```python
from build123d import *

# Parameters (mm, degrees)
SKETCH1_W           = 64
SKETCH1_H           = 76
TOP_DEPTH           = 2
SKETCH2_W           = 59.8
SKETCH2_H           = 71.8
BOSS_EXTRUDE2_DEPTH = 3
SKETCH3_W           = 10.5
SKETCH3_H           = 10.5
CUT_EXTRUDE1_DEPTH  = 6
SKETCH10_W          = 25.7
SKETCH10_H          = 27
CUT_EXTRUDE8_DEPTH  = 3
SKETCH11_W          = 7
SKETCH11_H          = 8
CUT_EXTRUDE9_DEPTH  = 1
SKETCH6_W           = 30
SKETCH6_H           = 25.4
CUT_EXTRUDE4_DEPTH  = 6
SKETCH7_R           = 1.15
BOSS_EXTRUDE3_DEPTH = 4.7
SKETCH8_W           = 40.8
SKETCH8_H           = 30.6
CUT_EXTRUDE6_DEPTH  = 4.7
SKETCH9_W           = 6.8
SKETCH9_H           = 15
CUT_EXTRUDE7_DEPTH  = 4.7
FILLET2_R           = 20
FILLET3_START       = 0.3
FILLET3_DEPTH       = 5.7
FILLET3_START_2     = 1
FILLET3_2_DEPTH     = 11
SKETCH14_R          = 1.15
BOSS_EXTRUDE4_DEPTH = 4.5
SKETCH12_W          = 11.9
SKETCH12_H          = 8
CUT_EXTRUDE10_DEPTH = 4
FILLET4_R           = 20
FILLET5_R           = 5


with BuildPart() as part:
    # Sketch1 → Top (new body)
    with BuildSketch(Plane(origin=(0, 0, 0), x_dir=(1, 0, 0), z_dir=(0, 1, 0))):
        Rectangle(SKETCH1_W, SKETCH1_H)
    extrude(amount=TOP_DEPTH)

    # Sketch2 → Boss-Extrude2 (add)
    with BuildSketch(Plane(origin=(0, 2, 0), x_dir=(1, 0, 0), z_dir=(0, 1, 0))):
        Rectangle(SKETCH2_W, SKETCH2_H)
    extrude(amount=BOSS_EXTRUDE2_DEPTH)

    # Sketch3 → Cut-Extrude1 (cut)
    with BuildSketch(Plane(origin=(0, 5, 0), x_dir=(1, 0, 0), z_dir=(0, 1, 0))):
        with Locations((-14.15, 20.15)):
            Rectangle(SKETCH3_W, SKETCH3_H)
    extrude(amount=-CUT_EXTRUDE1_DEPTH, mode=Mode.SUBTRACT)

    # Sketch10 → Cut-Extrude8 (cut)
    with BuildSketch(Plane(origin=(0, 5, 0), x_dir=(1, 0, 0), z_dir=(0, 1, 0))):
        with Locations((-14.15, 20.15)):
            Rectangle(SKETCH10_W, SKETCH10_H)
    extrude(amount=-CUT_EXTRUDE8_DEPTH, mode=Mode.SUBTRACT)

    # Sketch11 → Cut-Extrude9 (cut)
    with BuildSketch(Plane(origin=(0, 2, 0), x_dir=(1, 0, 0), z_dir=(0, 1, 0))):
        with Locations((-22.9, 20.15)):
            Rectangle(SKETCH11_W, SKETCH11_H)
        with Locations((-5.4, 20.15)):
            Rectangle(SKETCH11_W, SKETCH11_H)
    extrude(amount=-CUT_EXTRUDE9_DEPTH, mode=Mode.SUBTRACT)

    # Sketch6 → Cut-Extrude4 (cut)
    with BuildSketch(Plane(origin=(0, 5, 0), x_dir=(1, 0, 0), z_dir=(0, 1, 0))):
        with Locations((6.6, -17.5)):
            Rectangle(SKETCH6_W, SKETCH6_H)
    extrude(amount=-CUT_EXTRUDE4_DEPTH, mode=Mode.SUBTRACT)

    # Sketch7 → Boss-Extrude3 (add)
    with BuildSketch(Plane(origin=(0, 5, 0), x_dir=(1, 0, 0), z_dir=(0, 1, 0))):
        with Locations((-11.5, -4.5)):
            Circle(SKETCH7_R)
        with Locations((-11.5, -30.5)):
            Circle(SKETCH7_R)
        with Locations((24.7, -30.5)):
            Circle(SKETCH7_R)
        with Locations((24.7, -4.5)):
            Circle(SKETCH7_R)
    extrude(amount=-BOSS_EXTRUDE3_DEPTH)

    # Sketch8 → Cut-Extrude6 (cut)
    with BuildSketch(Plane(origin=(0, 5, 0), x_dir=(1, 0, 0), z_dir=(0, 1, 0))):
        with Locations((6.6, -17.5)):
            Rectangle(SKETCH8_W, SKETCH8_H)
    extrude(amount=-CUT_EXTRUDE6_DEPTH, mode=Mode.SUBTRACT)

    # Sketch9 → Cut-Extrude7 (cut)
    with BuildSketch(Plane(origin=(0, 5, 0), x_dir=(1, 0, 0), z_dir=(0, 1, 0))):
        with Locations((6.6, 5.3)):
            Rectangle(SKETCH9_W, SKETCH9_H)
    extrude(amount=-CUT_EXTRUDE7_DEPTH, mode=Mode.SUBTRACT)

    # Fillet2
    # the kernel refuses this fillet: 20 mm, written as the material it adds along each edge
    with BuildSketch(Plane(origin=(3.2, 0.3, -12.8), x_dir=(0, 0, 1), z_dir=(1, 0, 0))) as fillet2_piece_1:
        with BuildLine():
            CenterArc((12.880605576, -20), FILLET2_R, 90, 40.093007985)
            Line((0, -4.7), (0, 0))
            Line((0, 0), (12.880605576, 0))
        make_face()
    extrude(amount=6.8)

    # Fillet3: read off the stored shape, not the designer's step
    # Fillet3 outline → Fillet3 (cut)
    with BuildSketch(Plane(origin=(0, 0, 0), x_dir=(1, 0, 0), z_dir=(0, 1, 0)).offset(FILLET3_START)):
        with BuildLine():
            ThreePointArc((15, -2.2), (11.464466094, -0.735533906), (10, 2.8))
            Line((10, 2.8), (10, -2.2))
            Line((10, -2.2), (15, -2.2))
        make_face()
        with BuildLine():
            ThreePointArc((3.2, 2.8), (1.735533906, -0.735533906), (-1.8, -2.2))
            Line((-1.8, -2.2), (3.2, -2.2))
            Line((3.2, -2.2), (3.2, 2.8))
        make_face()
    extrude(amount=FILLET3_DEPTH, mode=Mode.SUBTRACT)

    # Fillet3 2 outline → Fillet3 2 (add)
    with BuildSketch(Plane.YZ.offset(FILLET3_START_2)):
        with BuildLine():
            Line((0.3, 0.080605576), (0.3, -2.8))
            Line((0.3, -2.8), (0.508534377, -2.8))
            ThreePointArc((0.508534377, -2.8), (0.35220172, -1.363466364), (0.3, 0.080605576))
        make_face()
    extrude(amount=FILLET3_2_DEPTH)

    # Sketch14 → Boss-Extrude4 (add)
    with BuildSketch(Plane(origin=(0, 0.3, 0), x_dir=(1, 0, 0), z_dir=(0, 1, 0))):
        with Locations(Location((-11.5, -4.5, 0), (0, 0, 270))):
            Circle(SKETCH14_R)
        with Locations(Location((24.7, -4.5, 0), (0, 0, 90))):
            Circle(SKETCH14_R)
        with Locations(Location((24.7, -30.5, 0), (0, 0, 270))):
            Circle(SKETCH14_R)
        with Locations(Location((-11.5, -30.5, 0), (0, 0, 90))):
            Circle(SKETCH14_R)
    extrude(amount=BOSS_EXTRUDE4_DEPTH)

    # Sketch12 → Cut-Extrude10 (cut)
    with BuildSketch(Plane(origin=(0, 5, 0), x_dir=(1, 0, 0), z_dir=(0, 1, 0))):
        with Locations((4.05, 20.15)):
            Rectangle(SKETCH12_W, SKETCH12_H)
    extrude(amount=-CUT_EXTRUDE10_DEPTH, mode=Mode.SUBTRACT)

    # Fillet4
    # the kernel refuses this fillet: 20 mm, written as the material it adds along each edge
    with BuildSketch(Plane(origin=(10, 1, -54.15), x_dir=(-1, 0, 0), z_dir=(0, 0, 1))) as fillet4_piece_1_section:
        with BuildLine():
            CenterArc((12, -20), FILLET4_R, 90, 36.869897646)
            Line((0, -4), (0, 0))
            Line((0, 0), (12, 0))
        make_face()
    fillet4_piece_1 = extrude(amount=38, mode=Mode.PRIVATE)
    fillet4_piece_1 = split(fillet4_piece_1, bisect_by=Plane(origin=(10, 1, -35.9), z_dir=(0, 0, 1)), keep=Keep.TOP, mode=Mode.PRIVATE)
    add(fillet4_piece_1)

    # Fillet5
    fillet5_edges = [part.edges().sort_by_distance(p)[0] for p in [
        (-1.3, 3.5, -24.15),
        (-1.3, 3.5, -16.15),
    ]]
    fillet(fillet5_edges, radius=FILLET5_R)


solid = part.part
```
The listing builds one solid part. Answer for the finished solid, in the listing's coordinates (mm). A direction names the side the tool comes from. Coordinates: 2 decimals unless noted, no trailing zeros. Loops run counter-clockwise (first coordinate to the right, second up) from the corner with the lowest first, then second, coordinate; pieces in that order, holes last. Notation, with made-up numbers: (27.5, 41.25) - (51.5, 41.25) arc R21 ccw to (51.5, 74.25) - close; hole circle Ø6 at (70.25, 62.5). An arc over 180 degrees is marked (long way). Use a Markdown table: item, result. Add a question column.
1) Find the intervals of material crossed by line 1 (X direction, y = 3.7, z = -10.5); line 2 (Z direction, x = -2.5, y = 2.7); line 3 (X direction, y = 2.6, z = -32.5), in increasing order.
2) For faces 1 (the flat face through (-5, 1, -20)), 2 (the flat face through (0, 1, 38)), 3 (the flat face through (-14, 1, -14.9)), 4 (the flat face through (0, 3, 35.9)), determine the directions among +Z, -Z, +X, -X, +Y, -Y from which every point of the face is accessible in a straight line to the end or side of a thin tool.
3) The part is cut by section C-C, the plane y = 3.5. Give the vertices of the cut face in (x, z), and give its area (3 significant figures).
4) Given pin 1 (2.5 mm diameter, centred on x = -11, z = 5, fed in from +Y); pin 2 (1.3 mm diameter, centred on y = 3, z = -6, fed in from -X); pin 3 (2 mm diameter, centred on x = 18, y = 4.5, fed in from +Z), each flat-ended and moving along its own axis, determine where each tip first touches the part or whether it passes through.
5) The part is cut by section D-D, the plane x = 24.7. Give the vertices of the cut face in (y, z), and give its area (3 significant figures).
6) The part is cut by section B-B, the plane z = -22. Give the vertices of the cut face in (x, y), and give its area (3 significant figures).
7) The part is cut by section A-A, the plane x = -4. Give the vertices of the cut face in (y, z), and give its area (3 significant figures).
Here are the results:
| question | item | result |
|---|---|---|
| 1 | line 1 | x = -29.9 to -27, -1.3 to 3.2, 10 to 29.9 |
| 1 | line 2 | z = -35.9 to -33.65, -6.65 to 2.2, 32.8 to 35.9 |
| 1 | line 3 | x = -29.9 to -27, -1.3 to 29.9 |
| 2 | face 1 | +Y |
| 2 | face 2 | +Z, +X, -X, +Y, -Y |
| 2 | face 3 | +Y, -Y |
| 2 | face 4 | +Z, +X, -X, +Y |
| 3 | outline | (-29.9, -35.9) - (29.9, -35.9) - (29.9, 35.9) - (-29.9, 35.9) - close; circle Ø2.3 at (-11.5, 4.5); circle Ø2.3 at (-11.5, 30.5); circle Ø2.3 at (24.7, 4.5); circle Ø2.3 at (24.7, 30.5); hole (-27, -33.65) - (-1.3, -33.65) - (-1.3, -29.15) arc R5 cw to (3.7, -24.15) - (7.68, -24.15) - (7.68, -16.15) - (3.7, -16.15) arc R5 cw to (-1.3, -11.15) - (-1.3, -6.65) - (-27, -6.65) - close; hole (-13.8, 2.2) - (-1.8, 2.2) arc R5 cw to (3.2, -2.8) - (3.2, -10.77) - (10, -10.77) - (10, -2.8) arc R5 cw to (15, 2.2) - (27, 2.2) - (27, 32.8) - (-13.8, 32.8) - close |
| 3 | area | 2,190 mm^2 |
| 4 | pin 1 | stops at y = 4.8 |
| 4 | pin 2 | stops at x = -29.9 |
| 4 | pin 3 | stops at z = 35.9 |
| 5 | outline | (0, -38) - (2, -38) - (2, -35.9) - (5, -35.9) - (5, 2.2) - (0.3, 2.2) - (0.3, 3.35) - (4.8, 3.35) - (4.8, 5.65) - (0.3, 5.65) - (0.3, 29.35) - (4.8, 29.35) - (4.8, 31.65) - (0.3, 31.65) - (0.3, 32.8) - (5, 32.8) - (5, 35.9) - (2, 35.9) - (2, 38) - (0, 38) - close |
| 5 | area | 244 mm^2 |
| 6 | outline | (-32, 0) - (-19.4, 0) - (-19.4, 1) - (-26.4, 1) - (-26.4, 2) - (-27, 2) - (-27, 5) - (-29.9, 5) - (-29.9, 2) - (-32, 2) - close; (-8.9, 0) - (32, 0) - (32, 2) - (29.9, 2) - (29.9, 5) - (10, 5) arc R20 cw to (-2, 1) - (-8.9, 1) - close |
| 6 | area | 165 mm^2 |
| 7 | outline | (0, -38) - (2, -38) - (2, -35.9) - (5, -35.9) - (5, -33.65) - (2, -33.65) - (2, -24.15) - (1, -24.15) - (1, -16.15) - (2, -16.15) - (2, -6.65) - (5, -6.65) - (5, 2.2) - (0.3, 2.2) - (0.3, 4.8) - (0, 4.8) - close; (0, 30.2) - (0.3, 30.2) - (0.3, 32.8) - (5, 32.8) - (5, 35.9) - (2, 35.9) - (2, 38) - (0, 38) - close |
| 7 | area | 127 mm^2 |
